For this review, take the finished solid that the model builds, in its own axes (mm). A direction names the side the tool comes from. Round coordinates to 2 decimals unless told otherwise and drop trailing zeros. Write each loop counter-clockwise with the first axis right and the second up, starting at its lowest first coordinate (ties: lowest second). Pieces come first, ordered by that corner, then holes. Notation, with made-up numbers: M 85.5,26.25 L 116.5,26.25 A28 ccw 116.5,47.25 Z; hole C 12.25,23.25 d10. An arc over 180 degrees is marked long. Use one line per item in the form item = value. Start each with the question number.
Item 1: For P1, Ø6, axis at y = -10, z = 0, coming from the -X side; P2, Ø12, axis at x = -170.5, y = 17.5, coming from the +Z side; P3, Ø3, axis at x = -24, y = 14, coming from the +Z side, all flat-tipped, find the tip position at first contact; note any pin that passes through.
Item 2: Draft analysis for pull direction Z (two halves, no side actions). For faces 1 (the cylindrical face through (-179.86, -13.32, 0.74)), 2 (the flat face through (-73, 0, 21)), 3 (the flat face through (-150, 6, 17)), 4 (the conical face through (-168.312, -9.502, 0.317)), state which applies: released by +Z, released by -Z, zero draft, split by the parting line, or undercut.
Item 3: Add section B-B (x = -137.5). State the section outline as (y, z) points, and give its area (3 significant figures).
Item 4: For line 1 (Y direction, x = -173, z = 0); line 2 (Z direction, x = -180, y = 10); line 3 (Z direction, x = -125, y = -0.5), list the stretches that pass through material, from the lowest coordinate up. Write a range as [from, to].
Item 5: For faces 5 (the cylindrical face through (-65.252, 19.961, 10.382)), 6 (the cylindrical face through (-64, 0, 22)), 7 (the flat face through (0, 0, 0)), list the 3-axis set-ups (+Z, -Z, +X, -X, +Y, -Y) from which the entire face can be reached by the end or side of a thin tool; tool diameter is ignored.
Item 6: Add section C-C (x = -32.5). State the section outline as (y, z) points.
from build123d import *

# Parameters (mm, degrees)
FASE1_SIZE                      = 2
FASE1_SIZE2                     = 0.535898385
FASE1_PART_2_SIZE               = 2
FASE1_PART_2_SIZE2              = 0.535898385
FASE1_PART_3_SIZE               = 2
FASE1_PART_3_SIZE2              = 0.535898385
SCHNITT_LINEAR_AUSTRAGEN1_DEPTH = 5.5
M8_GEWINDEBOHRUNG1_D            = 6.8
M8_GEWINDEBOHRUNG1_DEPTH        = 20
M8_GEWINDEBOHRUNG1_TIP          = 2.042926105
FASE2_SIZE                      = 2
FASE2_SIZE2                     = 0.535898385
SCHNITT_LINEAR_AUSTRAGEN2_DEPTH = 1.5


with BuildPart() as part:
    # Skizze1 → Rotation1 (revolve)
    with BuildSketch(Plane.XY, mode=Mode.PRIVATE) as rotation1_sk:
        Polygon((-85, 22.5), (-70, 22.5), (-47, 22.5), (-47, 27.5), (0, 27.5), (0, 0), (-190, 0), (-190, 20), (-110, 20), (-110, 21), (-85, 21), align=None)
    revolve(rotation1_sk.sketch.rotate(Axis((-55.076928245, 0, 0), (1, 0, 0)), 90), axis=Axis((-55.076928245, 0, 0), (1, 0, 0)))  # turned: the seam where the file's is

    # Fase1
    fase1_edges = [part.edges().sort_by_distance(p)[0] for p in [
        (-47, 0, -27.5),
    ]]
    fase1_side = [part.faces().sort_by_distance(p)[0] for p in [
        (-23.5, 0, -27.5),
    ]]
    chamfer(fase1_edges, length=FASE1_SIZE, length2=FASE1_SIZE2, reference=fase1_side[0])

    # Fase1 part 2
    fase1_part_2_edges = [part.edges().sort_by_distance(p)[0] for p in [
        (-85, 0, -22.5),
    ]]
    fase1_part_2_side = [part.faces().sort_by_distance(p)[0] for p in [
        (-66, 0, -22.5),
    ]]
    chamfer(fase1_part_2_edges, length=FASE1_PART_2_SIZE, length2=FASE1_PART_2_SIZE2, reference=fase1_part_2_side[0])

    # Fase1 part 3
    fase1_part_3_edges = [part.edges().sort_by_distance(p)[0] for p in [
        (-110, 0, -21),
    ]]
    fase1_part_3_side = [part.faces().sort_by_distance(p)[0] for p in [
        (-97.5, 0, -21),
    ]]
    chamfer(fase1_part_3_edges, length=FASE1_PART_3_SIZE, length2=FASE1_PART_3_SIZE2, reference=fase1_part_3_side[0])

    # Skizze2 → Schnitt-Linear austragen1 (cut)
    with BuildSketch(Plane.XY.offset(20)):
        with BuildLine():
            Line((-175.5, 6), (-124.5, 6))
            ThreePointArc((-124.5, 6), (-118.5, 0), (-124.5, -6))
            Line((-124.5, -6), (-175.5, -6))
            ThreePointArc((-175.5, -6), (-181.5, 0), (-175.5, 6))
        make_face()
    extrude(amount=-SCHNITT_LINEAR_AUSTRAGEN1_DEPTH, mode=Mode.SUBTRACT)

    # M8 Gewindebohrung1
    with Locations(Plane.ZY.offset(190)):
        with Locations((0, 10), (0, -10)):
            Hole(M8_GEWINDEBOHRUNG1_D / 2, depth=M8_GEWINDEBOHRUNG1_DEPTH)
            with Locations((0, 0, -(M8_GEWINDEBOHRUNG1_DEPTH + M8_GEWINDEBOHRUNG1_TIP / 2))):  # 118° drill point
                Cone(0, M8_GEWINDEBOHRUNG1_D / 2, M8_GEWINDEBOHRUNG1_TIP, mode=Mode.SUBTRACT)

    # Fase2
    fase2_edges = [part.edges().sort_by_distance(p)[0] for p in [
        (-190, 0, -20),
    ]]
    fase2_side = [part.faces().sort_by_distance(p)[0] for p in [
        (-150, 0, -20),
    ]]
    chamfer(fase2_edges, length=FASE2_SIZE, length2=FASE2_SIZE2, reference=fase2_side[0])

    # Skizze8 → Schnitt-Linear austragen2 (cut)
    with BuildSketch(Plane.XY.offset(22.5)):
        with BuildLine():
            Line((-83, 4), (-68, 4))
            ThreePointArc((-68, 4), (-64, 0), (-68, -4))
            Line((-68, -4), (-83, -4))
            Line((-83, -4), (-83, 4))
        make_face()
    extrude(amount=-SCHNITT_LINEAR_AUSTRAGEN2_DEPTH, mode=Mode.SUBTRACT)


solid = part.part
Calculated:
q1.P1 = -169.76
q1.P2 = 16.36
q1.P3 = 24.49
q2.face_1 = undercut
q2.face_2 = released by +Z
q2.face_3 = zero draft
q2.face_4 = undercut
q3.outline = M -6,14.5 L -6,19.08 A20 ccw long 6,19.08 L 6,14.5 Z
q3.area = 1,190 mm^2
q4.line_1 = [-20, -13.4], [-6.6, 6.6], [13.4, 20]
q4.line_2 = [-17.32, -3.4], [3.4, 17.32]
q4.line_3 = [-19.99, 14.5]
q5.face_5 = -X
q5.face_6 = +Z
q5.face_7 = +Z, -Z, +X, +Y, -Y
q6.outline = C 0,0 d55
